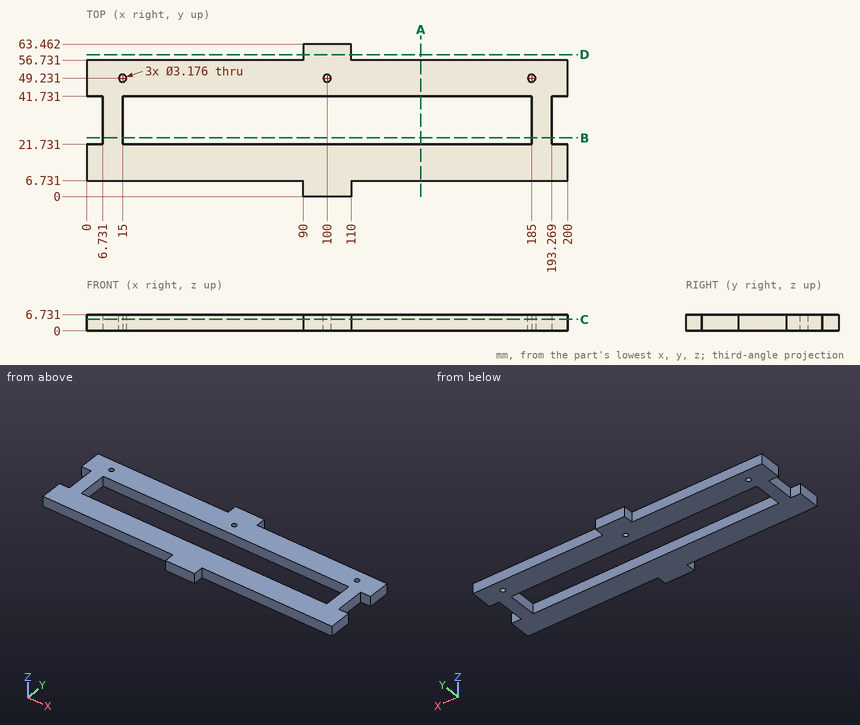
Verification items for this drawing (mm, ordinates from the low corner). Round coordinates to 2 decimals unless told otherwise and drop trailing zeros. Order: outer loops, then holes, each group sorted by start corner. A loop starts at its lowest first (then second) coordinate and runs counter-clockwise, first axis right, second up. Notation, with made-up numbers: (22.25, 1) -> (57.25, 1) arc R22 ccw to (57.25, 17) -> close; hole circle Ø2 at (-28.5, 87). An arc over 180 degrees is marked (long way). Use one line per item in the form item = value.
1. Go/stop test with flat-tipped pins: pin 1 (3.5 mm diameter, centred on x = 151, z = 4.5, fed in from +Y); pin 2 (2 mm diameter, centred on x = 139.5, z = 3, fed in from -Y); pin 3 (2 mm diameter, centred on y = 31.5, z = 2.5, fed in from -X); pin 4 (1.9 mm diameter, centred on x = 185, y = 49.231, fed in from +Z). Record where each tip stops, or that it passes through.
Working result:
pin_1 = 56.73
pin_2 = 6.73
pin_3 = 6.73
pin_4 = through
2. Scan lines: line 1 along Y through (x, z) = (76, 3.5); line 2 along X through (y, z) = (27, 6); line 3 along Y through (x, z) = (100, 4.5). Record each from-to range of solid material in increasing order. Write a range as from..to.
Working result:
line_1 = 6.73..21.73, 41.73..56.73
line_2 = 6.73..15, 185..193.27
line_3 = 0..21.73, 41.73..47.64, 50.82..63.46
3. Cross-section at B-B, the plane y = 24.5. Enter the section's corners in (x, z).
Working result:
outline = (6.73, 0) -> (15, 0) -> (15, 6.73) -> (6.73, 6.73) -> close; (185, 0) -> (193.27, 0) -> (193.27, 6.73) -> (185, 6.73) -> close
4. Cross-section at D-D, the plane y = 59. Enter the section's corners in (x, z).
Working result:
outline = (90, 0) -> (110, 0) -> (110, 6.73) -> (90, 6.73) -> close
5. Cross-section at A-A, the plane x = 139. Enter the section's corners in (y, z), plus the area to 3 significant figures.
Working result:
outline = (6.73, 0) -> (21.73, 0) -> (21.73, 6.73) -> (6.73, 6.73) -> close; (41.73, 0) -> (56.73, 0) -> (56.73, 6.73) -> (41.73, 6.73) -> close
area = 202 mm^2
6. Cross-section at C-C, the plane z = 4.75. Enter the section's corners in (x, y), plus the area to 3 significant figures.
Working result:
outline = (0, 6.73) -> (90, 6.73) -> (90, 0) -> (110, 0) -> (110, 6.73) -> (200, 6.73) -> (200, 21.73) -> (193.27, 21.73) -> (193.27, 41.73) -> (200, 41.73) -> (200, 56.73) -> (110, 56.73) -> (110, 63.46) -> (90, 63.46) -> (90, 56.73) -> (0, 56.73) -> (0, 41.73) -> (6.73, 41.73) -> (6.73, 21.73) -> (0, 21.73) -> close; hole circle Ø3.18 at (15, 49.23); hole (15, 21.73) -> (185, 21.73) -> (185, 41.73) -> (15, 41.73) -> close; hole circle Ø3.18 at (100, 49.23); hole circle Ø3.18 at (185, 49.23)
area = 6,580 mm^2
